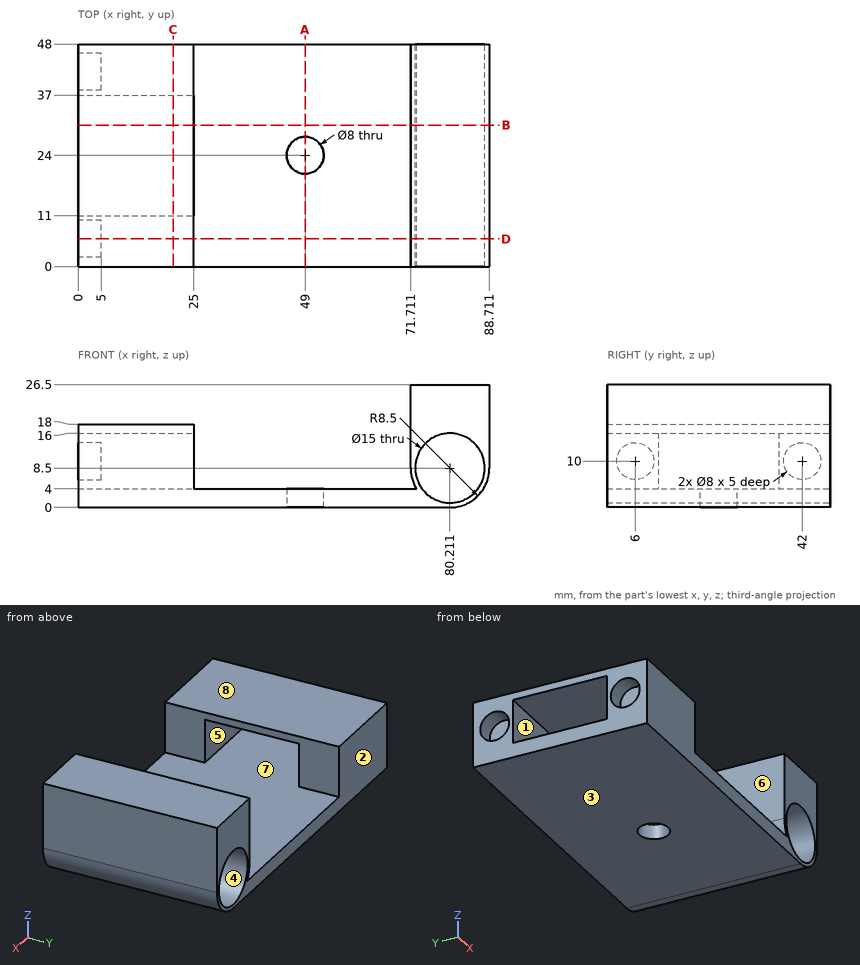
For this review, use the dimensioned drawing (mm, ordinates from the lowest corner) and the shaded views. A direction names the side the tool comes from. Coordinates: 2 decimals unless noted, no trailing zeros. Order: outer loops, then holes, each group sorted by start corner. A loop starts at its lowest first (then second) coordinate and runs counter-clockwise, first axis right, second up. Notation, with made-up numbers: (64, -8) - (85, -8) arc R9 cw to (85, 8) - close; hole circle Ø5 at (54, -19.5). An arc over 180 degrees is marked (long way). Answer as a JSON object with one key per item and string values. Group by question number.
1. We need section C-C on x = 20.5. State the section outline as (y, z) points.
2. Clearance check with flat-ended pins moving along their axes: P1, Ø14.5, axis at y = 32.5, z = 19.5, coming from the -X side; P2, Ø10.5, axis at x = 49, y = 24, coming from the +Z side; P3, Ø5, axis at y = 27.5, z = 11.5, coming from the -X side; P4, Ø7.5, axis at x = 11, y = 22, coming from the +Z side. State where each tip first meets the part, or that it passes through.
3. We need section B-B on y = 30.5. State the section outline as (x, z) points.
4. For probe 1 along Y at (x, z) = (3.4, 10); probe 2 along Y at (x, z) = (49, 1.9); probe 3 along X at (y, z) = (3, 13.5), list the stretches that pass through material, from the lowest coordinate up.
5. We need section D-D on y = 6. State the section outline as (x, z) points, then the cut area to 3 significant figures.
6. We need section A-A on x = 49. State the section outline as (y, z) points, then the cut area to 3 significant figures.
7. For the marked faces 5, 6, 7 and 8, list the 3-axis set-ups (+Z, -Z, +X, -X, +Y, -Y) from which the entire face can be reached by the end or side of a thin tool; tool diameter is ignored.
8. The part is to be moulded in two halves that separate along Z. For the marked faces 1, 2, 3 and 4, say which applies: pulls with the +Z half, pulls with the -Z half, needs draft (parallel to the pull), parting line crosses it, or undercut.
Final values:
{
 "1": {"outline": "(0, 0) - (48, 0) - (48, 18) - (0, 18) - close; hole (11, 4) - (37, 4) - (37, 16) - (11, 16) - close"},
 "2": {"P1": "x = 0", "P2": "z = 4", "P3": "x = 71.71", "P4": "z = 18"},
 "3": {"outline": "(0, 0) - (80.21, 0) arc R8.5 ccw to (88.71, 8.5) - (88.71, 26.5) - (71.71, 26.5) - (71.71, 8.5) arc R8.5 ccw to (73, 4) - (0, 4) - close; (0, 16) - (25, 16) - (25, 18) - (0, 18) - close; hole circle Ø15 at (80.21, 8.5)"},
 "4": {"probe 1": "0 to 2, 10 to 11, 37 to 38, 46 to 48", "probe 2": "0 to 20, 28 to 48", "probe 3": "0 to 25, 71.71 to 74.62, 85.8 to 88.71"},
 "5": {"outline": "(0, 0) - (80.21, 0) arc R8.5 ccw to (88.71, 8.5) - (88.71, 26.5) - (71.71, 26.5) - (71.71, 8.5) arc R8.5 ccw to (73, 4) - (25, 4) - (25, 18) - (0, 18) - (0, 14) - (5, 14) - (5, 6) - (0, 6) - close; hole circle Ø15 at (80.21, 8.5)", "area": "853 mm²"},
 "6": {"outline": "(0, 0) - (20, 0) - (20, 4) - (0, 4) - close; (28, 0) - (48, 0) - (48, 4) - (28, 4) - close", "area": "160 mm²"},
 "7": {"face 5": "-X", "face 6": "+Z, +Y, -Y", "face 7": "none", "face 8": "+Z, -X, +Y, -Y"},
 "8": {"face 1": "undercut", "face 2": "needs draft", "face 3": "pulls with the -Z half", "face 4": "undercut"}
}
